```python
from build123d import *

# Parameters (mm, degrees)
F0_W     = 90
F0_H     = 45
F1_DEPTH = 120
F2_T     = -8
F4_DEPTH = 8
F6_DEPTH = 120
F7_R     = 2
F8_R     = 1


# Not quite as in the source:
# - a feature names something its author has since deleted; it is built from what else it names


with BuildPart() as f1:
    # F0 (on Top) → F1 (new body)
    with BuildSketch(Plane.XY):
        Rectangle(F0_W, F0_H)
    extrude(amount=F1_DEPTH)

    # F2
    f2_openings = [f1.faces().sort_by_distance(p)[0] for p in [
        (0, 0, 120),
        (0, -22.5, 60),
        (0, 0, 0),
    ]]
    offset(amount=F2_T, openings=f2_openings)

    # F3 (on face) → F4 (cut, through all)
    with BuildSketch(Plane(origin=(0, 22.5, 0), x_dir=(-1, 0, 0), z_dir=(0, 1, 0))):
        with BuildLine():
            Line((-32, 20), (-32, 0))
            Line((-32, 0), (-28, 0))
            Line((-28, 0), (-28, 20))
            ThreePointArc((-28, 20), (-30, 22), (-32, 20))
        make_face()
        with BuildLine():
            Line((-8, 20), (-8, 0))
            Line((-8, 0), (-4, 0))
            Line((-4, 0), (-4, 20))
            ThreePointArc((-4, 20), (-6, 22), (-8, 20))
        make_face()
        with BuildLine():
            Line((12, 20), (12, 0))
            Line((12, 0), (16, 0))
            Line((16, 0), (16, 20))
            ThreePointArc((16, 20), (14, 22), (12, 20))
        make_face()
        with BuildLine():
            Line((31, 20), (31, 0))
            Line((31, 0), (35, 0))
            Line((35, 0), (35, 20))
            ThreePointArc((35, 20), (33, 22), (31, 20))
        make_face()
        with BuildLine():
            Line((35, 120), (31, 120))
            Line((31, 120), (31, 100))
            ThreePointArc((31, 100), (33, 98), (35, 100))
            Line((35, 100), (35, 120))
        make_face()
        with BuildLine():
            Line((16, 120), (12, 120))
            Line((12, 120), (12, 100))
            ThreePointArc((12, 100), (14, 98), (16, 100))
            Line((16, 100), (16, 120))
        make_face()
        with BuildLine():
            Line((-4, 120), (-8, 120))
            Line((-8, 120), (-8, 100))
            ThreePointArc((-8, 100), (-6, 98), (-4, 100))
            Line((-4, 100), (-4, 120))
        make_face()
        with BuildLine():
            Line((-28, 120), (-32, 120))
            Line((-32, 120), (-32, 100))
            ThreePointArc((-32, 100), (-30, 98), (-28, 100))
            Line((-28, 100), (-28, 120))
        make_face()
    extrude(amount=-F4_DEPTH, mode=Mode.SUBTRACT)

    # F5 (on face) → F6 (join, through all)
    with BuildSketch(Plane(origin=(0, 0, 0), x_dir=(1, 0, 0), z_dir=(0, 0, -1))):
        Polygon((-40, -22.5), (-45, -22.5), (-41, -37.5), (-36, -37.5), align=None)
        Polygon((-22, -22.5), (-27, -22.5), (-16.3333333333, -62.5), (-11.3333333333, -62.5), align=None)
        Polygon((8.6666666667, -62.5), (-2, -22.5), (-7, -22.5), (3.6666666667, -62.5), align=None)
        Polygon((28.6666666667, -62.5), (18, -22.5), (13, -22.5), (23.6666666667, -62.5), align=None)
        Polygon((45, -22.5), (40, -22.5), (50.6666666667, -62.5), (55.6666666667, -62.5), align=None)
    extrude(amount=-F6_DEPTH)

    # F7
    f7_edges = [f1.edges().sort_by_distance(p)[0] for p in [
        (55.666667, 62.5, 60),
        (50.666667, 62.5, 60),
        (-16.333333, 62.5, 60),
        (3.666667, 62.5, 60),
        (-11.333333, 62.5, 60),
        (-36, 37.5, 60),
        (-41, 37.5, 60),
        (23.666667, 62.5, 60),
        (28.666667, 62.5, 60),
        (8.666667, 62.5, 60),
    ]]
    fillet(f7_edges, radius=F7_R)

    # F8
    f8_edges = [f1.edges().sort_by_distance(p)[0] for p in [
        (-45, -22.5, 60),
        (-37, -22.5, 60),
        (37, -22.5, 60),
        (45, -22.5, 60),
    ]]
    fillet(f8_edges, radius=F8_R)


solid = f1.part
```
CAD build for the part. Positions are in the model's coordinates, mm. A direction names the side the tool comes from. Round coordinates to 2 decimals unless told otherwise and drop trailing zeros. Order: outer loops, then holes, each group sorted by start corner. A loop starts at its lowest first (then second) coordinate and runs counter-clockwise, first axis right, second up. Notation, with made-up numbers: (-7.75, 89) -> (28.25, 89) arc R20 ccw to (28.25, 97) -> close; hole circle Ø6 at (-38, 65.5). An arc over 180 degrees is marked (long way). Write item = value, one per line.
(1) Drill centre lines: L1, parallel to X at y = -17.5, z = 70; L2, parallel to X at y = 32, z = 81.5; L3, parallel to X at y = 48, z = 44.5. Where is each one in solid material? Low to high.
Answers follow:
L1 = -45 to -37, 37 to 45
L2 = -42.47 to -37.47, -24.47 to -19.47, -4.47 to 0.53, 15.53 to 20.53, 42.53 to 47.53
L3 = -20.2 to -15.2, -0.2 to 4.8, 19.8 to 24.8, 46.8 to 51.8
(2) 3-axis set-ups, long thin cutter, end or side, ignore diameter. For faces 1 (the flat face through (-35, 19, 110)), 2 (the flat face through (-12, 19, 10)), 3 (the flat face through (-35, 19, 10)), 4 (the flat face through (-1.937, 41.488, 59.16)), 5 (the flat face through (3.068, 41.505, 59.16)): which of +Z, -Z, +X, -X, +Y, -Y reach the whole face in a straight line?
Answers follow:
face_1 = +Z, +Y, -Y
face_2 = -Z, -Y
face_3 = -Z, +Y, -Y
face_4 = +Z, -Z, +Y
face_5 = +Z, -Z
(3) Cut at C-C (z = 103). State how many separate pieces and enclosed holes the cut face has, plus the area to 3 significant figures.
Answers follow:
separate_pieces = 5
enclosed_holes = 0
area = 2,050 mm²
(4) Pull direction Y, two halves, no side cores. Call faces 6 (the flat face through (41, -22.5, 59)), 7 (the flat face through (-16.932, 41.505, 59.16)), 8 (the flat face through (8, 19, 110)): +Y half, -Y half, draft (parallel to the pull), parting line (faces both ways), or undercut.
Answers follow:
face_6 = -Y half
face_7 = undercut
face_8 = draft
(5) Cut at B-B (x = -20.5). Write the cut outline in (y, z) (3 decimals).
Answers follow:
outline = (14.5, 0) -> (22.5, 0) -> (22.5, 120) -> (14.5, 120) -> close; (28.125, 0) -> (46.875, 0) -> (46.875, 120) -> (28.125, 120) -> close
(6) Cut at A-A (y = -3.5). Write the cut outline in (x, z).
Answers follow:
outline = (-45, 0) -> (-37, 0) -> (-37, 120) -> (-45, 120) -> close; (37, 0) -> (45, 0) -> (45, 120) -> (37, 120) -> close
(7) Flat gauge pins, fed straight in: P1, Ø2.5, axis at y = 20, z = 8.5, coming from the +X side; P2, Ø6, axis at x = 2, z = 20, coming from the -Y side; P3, Ø9, axis at y = 19.5, z = 110.5, coming from the +X side. Where does each tip first touch, or does it go through?
Answers follow:
P1 = 45
P2 = 14.5
P3 = 45.4
(8) Cut at D-D (y = 50). Write the cut outline in (x, z), plus the area to 3 significant figures.
Answers follow:
outline = (-19.67, 0) -> (-14.67, 0) -> (-14.67, 120) -> (-19.67, 120) -> close; (0.33, 0) -> (5.33, 0) -> (5.33, 120) -> (0.33, 120) -> close; (20.33, 0) -> (25.33, 0) -> (25.33, 120) -> (20.33, 120) -> close; (47.33, 0) -> (52.33, 0) -> (52.33, 120) -> (47.33, 120) -> close
area = 2,400 mm²
